Autodesk Inventor part; units mm, degrees
ref_plane "YZ Plane" through (0, 0, 0) normal (1, 0, 0) x (0, 1, 0)
ref_plane "XZ Plane" through (0, 0, 0) normal (0, 1, 0) x (-1, 0, 0)
ref_plane "XY Plane" through (0, 0, 0) normal (0, 0, 1) x (1, 0, 0)
sketch "スケッチ1" plane through (0, 0, 0) normal (0, 0, 1) x (1, 0, 0)
  line L0 (-44.3295, 0) -> (44.3295, 0) construction
  line L1 (0, 23.7122) -> (0, -23.7122) construction
  line L2 (-26.6016, -16.95) -> (26.6016, -16.95) construction
  line L3 (-23, 17.7575) -> (-23, -30.8175) construction
  line L4 (23, -30.8175) -> (23, 17.7575) construction
  line L5 (-31, 17.7575) -> (-31, -30.8175) construction
  line L6 (31, -30.8175) -> (31, 17.7575) construction
  circle A0 centre (-31, 0) radius 1.6
  circle A1 centre (-23, -16.95) radius 1.6
  circle A2 centre (23, -16.95) radius 1.6
  circle A3 centre (31, 0) radius 1.6
  line L7 (-29.5, 6.55) -> (29.5, 6.55)
  line L8 (29.5, 6.55) -> (29.5, -22.45)
  line L9 (29.5, -22.45) -> (-29.5, -22.45)
  line L10 (-29.5, -22.45) -> (-29.5, 6.55)
  circle A4 centre (-23, -16.95) radius 3.5
  circle A5 centre (-31, 0) radius 3.5
  circle A6 centre (23, -16.95) radius 3.5
  circle A7 centre (31, 0) radius 3.5
  line L11 (-31.5, 8.55) -> (31.5, 8.55)
  line L12 (-31.5, 8.55) -> (-31.5, -24.45)
  line L13 (31.5, 8.55) -> (31.5, -24.45)
  line L14 (-31.5, -24.45) -> (31.5, -24.45)
  line L15 (-23, -20.45) -> (23, -20.45)
  line L16 (-26.5, -22.45) -> (-26.5, -24.45)
  line L17 (26.5, -24.45) -> (26.5, -22.45)
  line L18 (-31.5, -14.45) -> (-29.5, -14.45)
  line L19 (-31.5, 3.5) -> (-29.5, 3.5)
  line L20 (29.5, 3.5) -> (31.5, 3.5)
  line L21 (29.5, -14.45) -> (31.5, -14.45)
  line L22 (-21.5, 8.55) -> (-21.5, 6.55)
  line L23 (23.5, 8.55) -> (23.5, 6.55)
  line L24 (-16.5, 8.55) -> (-16.5, -24.45)
  line L25 (-14.5, -24.45) -> (-14.5, 8.55)
  line L26 (16.5, 8.55) -> (16.5, -24.45)
  line L27 (14.5, -24.45) -> (14.5, 8.55)
  line L28 (-40.1456, -7.95) -> (40.1456, -7.95) construction
  line L29 (-1.5, 8.55) -> (-1.5, 10.55)
  line L30 (-1.5, 10.55) -> (-4.5, 10.55)
  line L31 (-4.5, 10.55) -> (-4.5, 11.75)
  line L32 (-4.5, 11.75) -> (4.5, 11.75)
  line L33 (4.5, 11.75) -> (4.5, 10.55)
  line L34 (4.5, 10.55) -> (1.5, 10.55)
  line L35 (1.5, 10.55) -> (1.5, 8.55)
  line L36 (-1.5, -24.45) -> (-1.5, -26.45)
  line L37 (-1.5, -26.45) -> (-4.5, -26.45)
  line L38 (-4.5, -26.45) -> (-4.5, -27.65)
  line L39 (-4.5, -27.65) -> (4.5, -27.65)
  line L40 (4.5, -27.65) -> (4.5, -26.45)
  line L41 (4.5, -26.45) -> (1.5, -26.45)
  line L42 (1.5, -26.45) -> (1.5, -24.45)
  point P0 (0, 0)
  point P1 (0, 0)
  point P2 (0, -16.95)
  point P3 (0, -22.45)
  point P4 (-31.5, 3.4641)
  point P5 (-31.5, -3.4641)
  point P6 (-26.3541, -17.95)
  point P7 (26.3541, -17.95)
  point P8 (31.5, -3.4641)
  point P9 (31.5, 3.4641)
  point P10 (29.5, -3.1623)
  point P11 (25.8723, -14.95)
  point P12 (-19.6459, -17.95)
  point P13 (19.6459, -17.95)
  point P14 (20.1277, -14.95)
  point P15 (-20.1277, -14.95)
  point P16 (-25.8723, -14.95)
  point P17 (-29.5, -3.1623)
  point P18 (29.5, 3.1623)
  point P19 (-29.5, 3.1623)
  point P20 (0, -7.95)
  point P21 (16.5, -22.45)
  point P22 (14.5, -22.45)
  point P23 (-14.5, -22.45)
  point P24 (-16.5, -22.45)
  point P25 (16.5, 6.55)
  point P26 (14.5, 6.55)
  point P27 (-14.5, 6.55)
  point P28 (-16.5, 6.55)
  point P29 (14.5, -20.45)
  point P30 (-14.5, -20.45)
  dimension "MOUNT_W" = 16.95
  dimension "d1" = 23
  dimension "d2" = 31
  dimension "d3" = 3.2
  dimension "d4" = 59
  dimension "d5" = 29
  dimension "d8" = 7
  dimension "d9" = 2
  dimension "d10" = 2
  dimension "d11" = 2
  dimension "d12" = 2
  dimension "d18" = 8
  dimension "d19" = 8
  dimension "d20" = 8
  dimension "d24" = 2
  dimension "d25" = 2
  dimension "d26" = 2
  dimension "d27" = 13
  dimension "d28" = 13
  dimension "d33" = 3
  dimension "d34" = 9
  dimension "d35" = 2
  dimension "d36" = 1.2
extrude "ベース" add sketch "スケッチ1" against normal blind 1.5 contours A0 L10 A5 | A0 L12 A5 L10 | L10 A5 L12 A0 | A0 L12 A5 | A5 L19 L10 | A4 | L10 L7 L24 L9 A5 | L10 L18 L12 A5 | L12 L19 A5 | L19 L12 L11 L22 L7 L10 | L10 L9 L16 L14 L12 L18 | L22 L11 L24 L7 | L9 L24 L14 L16 | L24 L11 L25 L7 | L7 L25 L15 L24 | L24 L15 L25 L9 | L9 L25 L14 L24 | L25 L11 L27 L7 | L7 L27 L15 L25 | L25 L15 L27 L9 | L9 L27 L14 L25 | L27 L11 L26 L7 | L7 L26 L15 L27 | L27 L15 L26 L9 | L9 L26 L14 L27 | L26 L11 L23 L7 | A6 | L7 L8 A7 L9 L26 | L9 L17 L14 L26 | L23 L11 L13 L20 L8 L7 | L9 L8 L21 L13 L14 L17 | L20 A7 L8 | L8 A7 L13 L21 | A7 L13 A3 L8 | L8 A3 A7 | L20 L13 A7 | L8 A3 L13 A7 | A7 L13 A3
extrude "囲い柱" add sketch "スケッチ1" along normal blind 12 contours L19 L12 L11 L22 L7 L10 | L10 L9 L16 L14 L12 L18 | L23 L11 L13 L20 L8 L7 | L9 L8 L21 L13 L14 L17
extrude "底上げ" add sketch "スケッチ1" along normal blind 5 contours L22 L11 L24 L7 | L9 L24 L14 L16 | L24 L11 L25 L7 | L7 L25 L15 L24 | L24 L15 L25 L9 | L9 L25 L14 L24 | L25 L11 L27 L7 | L9 L27 L14 L25 | L27 L11 L26 L7 | L7 L26 L15 L27 | L27 L15 L26 L9 | L9 L26 L14 L27 | L26 L11 L23 L7 | L9 L17 L14 L26
extrude "肉抜き" cut sketch "スケッチ1" against normal through all contours L7 L27 L15 L25 | L25 L15 L27 L9
extrude "輪ゴムタブ" add sketch "スケッチ1" along normal blind 5 and the other way blind 1.5 contours L29 L30 L31 L32 L33 L34 L35 L11 | L14 L42 L41 L40 L39 L38 L37 L36
fillet "フィレット1" radius 1.5 4 edges at (-31.5, 8.55, 5.25) (31.5, 8.55, 5.25) (-31.5, -24.45, 5.25) (31.5, -24.45, 5.25)
fillet "フィレット2" radius 0.5 15 edges at (-4.5, 11.75, 1.75) (-4.5, 10.55, 1.75) (4.5, 10.55, 1.75) (4.5, 11.75, 1.75) (1.5, 10.55, 1.75) (1.5, 8.55, 1.75) (-1.5, 10.55, 1.75) (-1.5, 8.55, 1.75) (-1.5, -26.45, 1.75) (-4.5, -26.45, 1.75) (-4.5, -27.65, 1.75) (4.5, -26.45, 1.75) (1.5, -24.45, 1.75) (4.5, -27.65, 1.75) (1.5, -26.45, 1.75)
equation "\"d5\" = BAT_W + CLEARANCE"
equation "\"d9\" = TAB_W"
equation "\"d10\" = d9"
equation "\"d11\" = d9"
equation "\"d12\" = d9"
equation "\"d18\" = d19"
equation "\"d20\" = d19"
equation "\"d26\" = d25"
equation "\"d28\" = d27"
equation "\"d22\" = TAB_H"
equation "\"BAT_L\" = 58"
equation "\"BAT_W\" = 28"
equation "\"CLEARANCE\" = 1"
equation "\"TAB_W\" = 2"
equation "\"TAB_H\" = 12"
properties part number "Battery-Holder-2x2"
For this review, take the finished solid that the model builds, in its own axes (mm). A direction names the side the tool comes from. Give positions to 0.01 mm unless a question says otherwise; leave off trailing zeros. Order: outer loops, then holes, each group sorted by start corner. A loop starts at its lowest first (then second) coordinate and runs counter-clockwise, first axis right, second up. Notation, with made-up numbers: (-12, 45) -> (6, 45) arc R18 ccw to (6, 70) -> close; hole circle Ø6 at (13.25, 88.5). An arc over 180 degrees is marked (long way). Write item = value, one per line.
1) We need section C-C, the plane z = 7. Give the boundary of the cut face in (x, y), and give its area (3 significant figures).
Findings:
outline = (-31.5, -22.95) arc R1.5 ccw to (-30, -24.45) -> (-26.5, -24.45) -> (-26.5, -22.45) -> (-29.5, -22.45) -> (-29.5, -14.45) -> (-31.5, -14.45) -> close; (-31.5, 3.5) -> (-29.5, 3.5) -> (-29.5, 6.55) -> (-21.5, 6.55) -> (-21.5, 8.55) -> (-30, 8.55) arc R1.5 ccw to (-31.5, 7.05) -> close; (23.5, 6.55) -> (29.5, 6.55) -> (29.5, 3.5) -> (31.5, 3.5) -> (31.5, 7.05) arc R1.5 ccw to (30, 8.55) -> (23.5, 8.55) -> close; (26.5, -24.45) -> (30, -24.45) arc R1.5 ccw to (31.5, -22.95) -> (31.5, -14.45) -> (29.5, -14.45) -> (29.5, -22.45) -> (26.5, -22.45) -> close
area = 98.3 mm^2
2) We need section A-A, the plane x = -23. Give the boundary of the cut face in (y, z), and give its area (3 significant figures).
Findings:
outline = (-24.45, -1.5) -> (-18.55, -1.5) -> (-18.55, 0) -> (-22.45, 0) -> (-22.45, 5) -> (-24.45, 5) -> close; (-15.35, -1.5) -> (8.55, -1.5) -> (8.55, 12) -> (6.55, 12) -> (6.55, 0) -> (-15.35, 0) -> close
area = 78.7 mm^2
3) Insertion check: pin 1 (3.5 mm diameter, centred on x = 22.5, z = 8.5, fed in from -Y); pin 2 (1 mm diameter, centred on y = 7.5, z = 9, fed in from +X); pin 3 (2 mm diameter, centred on x = -14, z = 0.5, fed in from +Y). Each pin has a flat end and moves straight along its axis. Give the tip position at first contact, or say it passes through.
Findings:
pin_1 = 6.55
pin_2 = 31.5
pin_3 = 8.55
4) Draft analysis for pull direction X (two halves, no side actions). For faces 4 (the face through (16, -24.45, 2)), 5 (the face through (-1.5, -25, 2)), 6 (the face through (-16.5, -8, 2)), state which applies: pulls with the +X half, pulls with the -X half, needs draft (parallel to the pull), parting line crosses it, or undercut.
Findings:
face_4 = needs draft
face_5 = pulls with the -X half
face_6 = undercut
5) We need section D-D, the plane y = -8. Give the boundary of the cut face in (x, z).
Findings:
outline = (-31.5, -1.5) -> (-14.5, -1.5) -> (-14.5, 5) -> (-16.5, 5) -> (-16.5, 0) -> (-31.5, 0) -> close; (14.5, -1.5) -> (31.5, -1.5) -> (31.5, 0) -> (16.5, 0) -> (16.5, 5) -> (14.5, 5) -> close
6) To check wall thickness, follow L1, parallel to X at y = 0, z = -0.3; L2, parallel to X at y = -20, z = 9.5; L3, parallel to Y at x = 7.5, z = 4.5. State the ranges of each line that lie inside material, in increasing order. Write a range as from..to.
Findings:
L1 = -34.5..-32.6, -29.4..-14.5, 14.5..29.4, 32.6..34.5
L2 = -31.5..-29.5, 29.5..31.5
L3 = -24.45..-22.45, 6.55..8.55
7) For faces 1 (the face through (-25, 6.55, 6)), 2 (the face through (-31, 3.5, 6)), 3 (the face through (0, 6.55, 2)), list the 3-axis set-ups (+Z, -Z, +X, -X, +Y, -Y) from which the entire face can be reached by the end or side of a thin tool; tool diameter is ignored.
Findings:
face_1 = +Z
face_2 = +Z, -X
face_3 = +Z, -Z
8) We need section B-B, the plane y = -16.95. Give the boundary of the cut face in (x, z).
Findings:
outline = (-31.5, -1.5) -> (-24.6, -1.5) -> (-24.6, 0) -> (-29.5, 0) -> (-29.5, 12) -> (-31.5, 12) -> close; (-21.4, -1.5) -> (-14.5, -1.5) -> (-14.5, 5) -> (-16.5, 5) -> (-16.5, 0) -> (-21.4, 0) -> close; (14.5, -1.5) -> (21.4, -1.5) -> (21.4, 0) -> (16.5, 0) -> (16.5, 5) -> (14.5, 5) -> close; (24.6, -1.5) -> (31.5, -1.5) -> (31.5, 12) -> (29.5, 12) -> (29.5, 0) -> (24.6, 0) -> close
